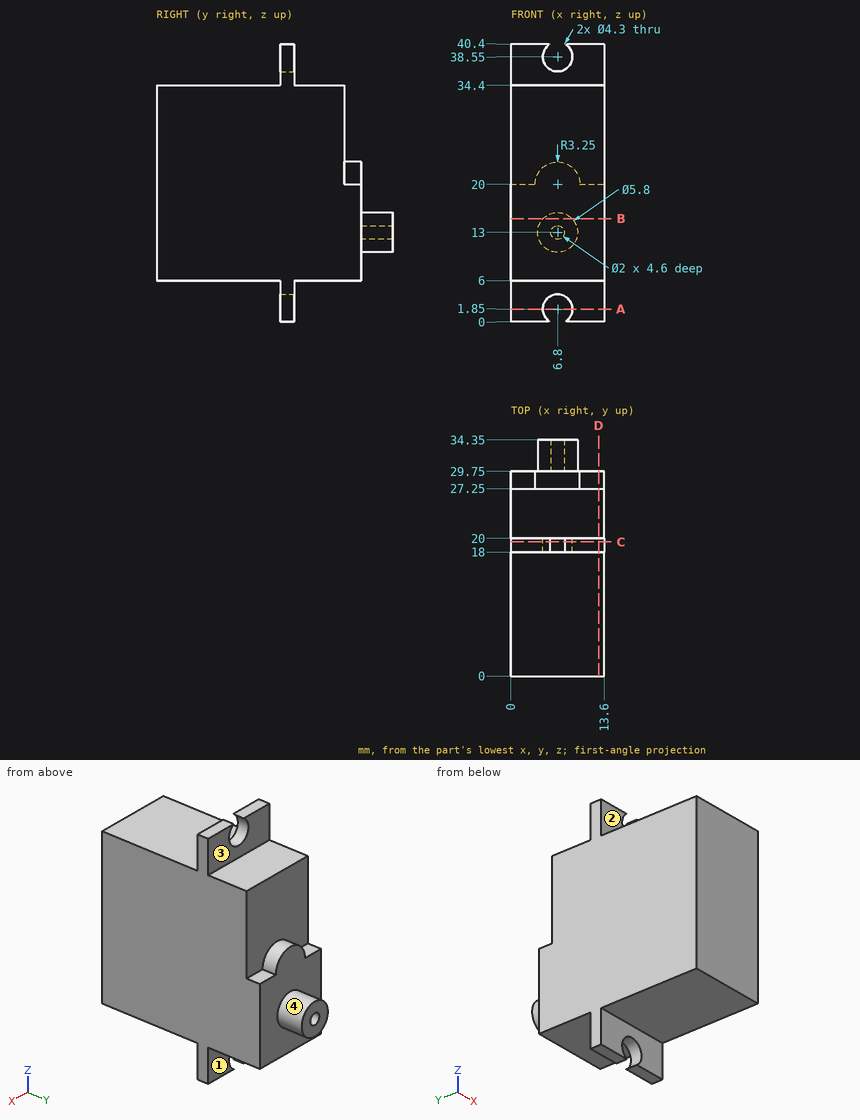
Part print with two shaded views. Sizes in mm from the minimum x, y, z corner. A direction names the side the tool comes from. Round coordinates to 2 decimals unless told otherwise and drop trailing zeros. Write each loop counter-clockwise with the first axis right and the second up, starting at its lowest first coordinate (ties: lowest second). Pieces come first, ordered by that corner, then holes. Notation, with made-up numbers: M 6,76.25 L 19,76.25 A17 ccw 19,98.25 Z; hole C 45.25,7 d4. An arc over 180 degrees is marked long. Put each result on its own line as item: value. Start each with the question number.
1) Pin check, flat tips, straight feed: pin 1 Ø6.5 at (x, z) = (5, 37) entering from +Y; pin 2 Ø1.6 at (x, z) = (6.8, 13) entering from +Y; pin 3 Ø2 at (x, y) = (7.5, 24.5) entering from +Z. Stop position of each tip, or through.
2) 3-axis set-ups, long thin cutter, end or side, ignore diameter. For the marked faces 1, 2, 3 and 4: which of +Z, -Z, +X, -X, +Y, -Y reach the whole face in a straight line?
3) Saw through at C-C, the plane y = 19.5. Write the cut outline in (x, z), and give its area (3 significant figures).
4) Saw through at B-B, the plane z = 15. Write the cut outline in (x, y).
5) Saw through at A-A, the plane z = 1.85. Write the cut outline in (x, y), and give its area (3 significant figures).
6) Saw through at D-D, the plane x = 12.75. Write the cut outline in (y, z), and give its area (3 significant figures).
7) Drill centre lines: probe 1 along X at (y, z) = (19.6, 38.55); probe 2 along X at (y, z) = (33, 13); probe 3 along Z at (x, y) = (3.25, 17). Where is each one in solid material? Low to high. Write a range as [from, to].
Resolved:
1. pin 1: y = 27.25
1. pin 2: y = 29.75
1. pin 3: z = 34.4
2. face 1: -Z, +X, -X, +Y
2. face 2: +Z, +X, -X, -Y
2. face 3: +Z, +X, -X, +Y
2. face 4: +Y
3. outline: M 0,0 L 5.7,0 A2.15 cw long 7.9,0 L 13.6,0 L 13.6,40.4 L 7.9,40.4 A2.15 cw long 5.7,40.4 L 0,40.4 Z
3. area: 521 mm²
4. outline: M 0,0 L 13.6,0 L 13.6,29.75 L 8.9,29.75 L 8.9,34.35 L 4.7,34.35 L 4.7,29.75 L 0,29.75 Z
5. outline: M 0,18 L 4.65,18 L 4.65,20 L 0,20 Z; M 8.95,18 L 13.6,18 L 13.6,20 L 8.95,20 Z
5. area: 18.6 mm²
6. outline: M 0,6 L 18,6 L 18,0 L 20,0 L 20,6 L 29.75,6 L 29.75,20 L 27.25,20 L 27.25,34.4 L 20,34.4 L 20,40.4 L 18,40.4 L 18,34.4 L 0,34.4 Z
6. area: 833 mm²
7. probe 1: [0, 4.65], [8.95, 13.6]
7. probe 2: [3.9, 5.8], [7.8, 9.7]
7. probe 3: [6, 34.4]
